```python
from build123d import *

# Parameters (mm, degrees)
SKETCH1_R           = 9
BOSS_EXTRUDE1_DEPTH = 68
SKETCH2_R           = 3.5
BOSS_EXTRUDE2_DEPTH = 7
BOSS_EXTRUDE3_DEPTH = 2
BOSS_EXTRUDE4_START = -6
BOSS_EXTRUDE4_DEPTH = 2


with BuildPart() as part:
    # Sketch1 → Boss-Extrude1 (new body)
    with BuildSketch(Plane.XY):
        Circle(SKETCH1_R)
    extrude(amount=BOSS_EXTRUDE1_DEPTH)

    # Sketch2 → Boss-Extrude2 (add)
    with BuildSketch(Plane.XY.offset(68)):
        with Locations((0, -4)):
            Circle(SKETCH2_R)
    extrude(amount=BOSS_EXTRUDE2_DEPTH)

    # Sketch4 → Boss-Extrude3 (add)
    with BuildSketch(Plane(origin=(0, 0, 9), x_dir=(-1, 0, 0), z_dir=(0, 0, -1))):
        Polygon((-12, 6.92820323), (-12, -6.92820323), (0, -13.856406461), (12, -6.92820323), (12, 6.92820323), (0, 13.856406461), align=None)
    extrude(amount=-BOSS_EXTRUDE3_DEPTH)

    # Sketch4<2> → Boss-Extrude4 (add)
    with BuildSketch(Plane(origin=(0, 0, 9), x_dir=(-1, 0, 0), z_dir=(0, 0, -1)).offset(BOSS_EXTRUDE4_START)):
        Polygon((-12, 6.92820323), (-12, -6.92820323), (0, -13.856406461), (12, -6.92820323), (12, 6.92820323), (0, 13.856406461), align=None)
    extrude(amount=BOSS_EXTRUDE4_DEPTH)


solid = part.part
```
Source: CAD feature listing. Evaluate the final solid. Frame: model axes, mm. A direction names the side the tool comes from. Round coordinates to 2 decimals unless told otherwise and drop trailing zeros. Loops run counter-clockwise (first coordinate to the right, second up) from the corner with the lowest first, then second, coordinate; pieces in that order, holes last.
1. Section query B-B on x = -9.75. Output: boundary loops of the cut face in (y, z).
2. Contact query for flat-ended pins moving along their axis: pin 1 (4 mm diameter, centred on x = 3, z = 13.5, fed in from -Y); pin 2 (7 mm diameter, centred on x = -5, y = 2, fed in from +Z); pin 3 (5 mm diameter, centred on x = 0, z = 26.5, fed in from -Y); pin 4 (12 mm diameter, centred on y = -7, z = 14, fed in from +X). Output: stop coordinate, or through.
3. Section query A-A on y = -10.5. Output: boundary loops of the cut face in (x, z), and give its area (3 significant figures).
4. Section query C-C on y = -4. Output: boundary loops of the cut face in (x, z).
5. Section query D-D on x = -5.5. Output: boundary loops of the cut face in (y, z).
6. Mould query, pull axis Z, two halves, no side actions, for faces 1 (the flat face through (5.92, 10.44, 14.01)), 2 (the flat face through (0, -4, 75)), 3 (the cylindrical face through (-1.172, 8.923, 11.986)). Classes: released by +Z, released by -Z, zero draft, split by the parting line, or undercut.
7. Ray query, L1, parallel to Z at x = 9.25, y = 8; L2, parallel to Z at x = -2.25, y = 6; L3, parallel to Y at x = -5.75, z = 23. Return the intervals inside material, ascending.
8. Access query for faces 4 (the flat face through (3, -9, 13)), 5 (the cylindrical face through (-1.172, 8.923, 41.129)), 6 (the cylindrical face through (-1.172, 8.923, 4.437)). Directions: +Z, -Z, +X, -X, +Y, -Y. A direction counts if a zero-diameter tool reaches every point of the face in a straight line with its end or side. Return the directions, or none.
Answers below:
1. outline: (-8.23, 9) - (8.23, 9) - (8.23, 11) - (-8.23, 11) - close; (-8.23, 13) - (8.23, 13) - (8.23, 15) - (-8.23, 15) - close
2. pin 1: stops at y = -13.28
2. pin 2: stops at z = 68
2. pin 3: stops at y = -9
2. pin 4: stops at x = 12
3. outline: (-5.81, 9) - (5.81, 9) - (5.81, 11) - (-5.81, 11) - close; (-5.81, 13) - (5.81, 13) - (5.81, 15) - (-5.81, 15) - close
3. area: 46.5 mm2
4. outline: (-12, 9) - (-8.06, 9) - (-8.06, 0) - (8.06, 0) - (8.06, 9) - (12, 9) - (12, 11) - (8.06, 11) - (8.06, 13) - (12, 13) - (12, 15) - (8.06, 15) - (8.06, 68) - (3.5, 68) - (3.5, 75) - (-3.5, 75) - (-3.5, 68) - (-8.06, 68) - (-8.06, 15) - (-12, 15) - (-12, 13) - (-8.06, 13) - (-8.06, 11) - (-12, 11) - close
5. outline: (-10.68, 9) - (-7.12, 9) - (-7.12, 0) - (7.12, 0) - (7.12, 9) - (10.68, 9) - (10.68, 11) - (7.12, 11) - (7.12, 13) - (10.68, 13) - (10.68, 15) - (7.12, 15) - (7.12, 68) - (-7.12, 68) - (-7.12, 15) - (-10.68, 15) - (-10.68, 13) - (-7.12, 13) - (-7.12, 11) - (-10.68, 11) - close
6. face 1: zero draft
6. face 2: released by +Z
6. face 3: undercut
7. L1: z = 9 to 11, 13 to 15
7. L2: z = 0 to 68
7. L3: y = -6.92 to 6.92
8. face 4: none
8. face 5: +Z
8. face 6: -Z
